Geometry: final body of the model. Coordinates: model frame, mm. Give positions to 0.01 mm unless a question says otherwise; leave off trailing zeros. Write each loop counter-clockwise with the first axis right and the second up, starting at its lowest first coordinate (ties: lowest second). Pieces come first, ordered by that corner, then holes.
Q1. Section A-A (z = -6). Return the cut outline in (x, y), plus the area to 3 significant figures.
Q2. Section B-B (x = -18). Return the cut outline in (y, z), plus the area to 3 significant figures.
Q3. Section C-C (y = -0.35). Return the cut outline in (x, z).
Q4. Pin query (flat end, axial travel): pin 1 Ø4.5 at (x, z) = (-36.5, 36.5) entering from +Y; pin 2 Ø0.8 at (x, y) = (7, -0.5) entering from +Z; pin 3 Ø0.8 at (y, z) = (-0.5, -15.5) entering from +X. Return the tip coordinate at first contact, or that it passes through.
Q5. Line query: line 1 (Z direction, x = 36.5, y = 0.75); line 2 (X direction, y = 0.55, z = -1). Output: solid intervals per line, ascending.
Q6. Section D-D (x = 36.5). Return the cut outline in (y, z), plus the area to 3 significant figures.
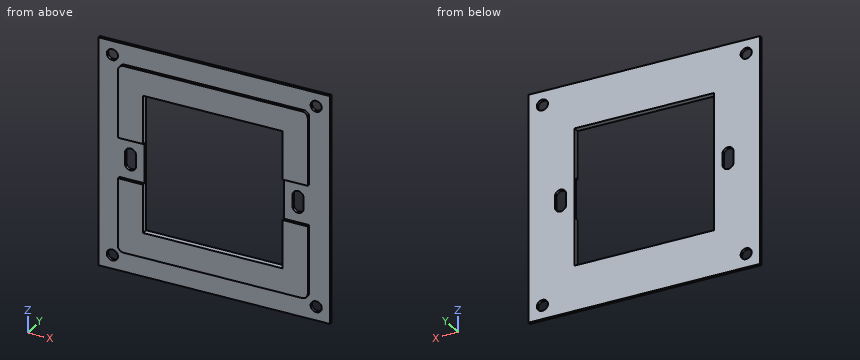
from build123d import *

# Parameters (mm, degrees)
SKETCH_1_W      = 83
SKETCH_1_H      = 83
SKETCH_1_R      = 2
SKETCH_1_W_2    = 50
SKETCH_1_H_2    = 50
EXTRUDE_1_DEPTH = 1
EXTRUDE_2_DEPTH = 1


with BuildPart() as part:
    # Эскиз1 → Бобышка-Вытянуть1 (new body)
    with BuildSketch(Plane(origin=(0, 0, 0), x_dir=(1, 0, 0), z_dir=(0, 1, 0))):
        Rectangle(SKETCH_1_W, SKETCH_1_H)
        with Locations((36.5, 36.5)):
            Circle(SKETCH_1_R, mode=Mode.SUBTRACT)
        with Locations((-36.5, 36.5)):
            Circle(SKETCH_1_R, mode=Mode.SUBTRACT)
        with Locations((-36.5, -36.5)):
            Circle(SKETCH_1_R, mode=Mode.SUBTRACT)
        with Locations((36.5, -36.5)):
            Circle(SKETCH_1_R, mode=Mode.SUBTRACT)
        with BuildLine():
            Line((28, 2), (28, -2))
            ThreePointArc((28, -2), (30, -4), (32, -2))
            Line((32, -2), (32, 2))
            ThreePointArc((32, 2), (30, 4), (28, 2))
        make_face(mode=Mode.SUBTRACT)
        Rectangle(SKETCH_1_W_2, SKETCH_1_H_2, mode=Mode.SUBTRACT)
        with BuildLine():
            Line((-32, 2), (-32, -2))
            ThreePointArc((-32, -2), (-30, -4), (-28, -2))
            Line((-28, -2), (-28, 2))
            ThreePointArc((-28, 2), (-30, 4), (-32, 2))
        make_face(mode=Mode.SUBTRACT)
    extrude(amount=EXTRUDE_1_DEPTH)

    # Эскиз2 → Бобышка-Вытянуть2 (add)
    with BuildSketch(Plane(origin=(0, 0, 0), x_dir=(1, 0, 0), z_dir=(0, 1, 0))):
        with BuildLine():
            Line((-25, -7.393137128), (-34, -7.393137128))
            Line((-34, -7.393137128), (-34, -32))
            ThreePointArc((-34, -32), (-33.414213562, -33.414213562), (-32, -34))
            Line((-32, -34), (32, -34))
            ThreePointArc((32, -34), (33.414213562, -33.414213562), (34, -32))
            Line((34, -32), (34, -7.393137128))
            Line((34, -7.393137128), (25, -7.393137128))
            Line((25, -7.393137128), (25, -25))
            Line((25, -25), (-25, -25))
            Line((-25, -25), (-25, -7.393137128))
        make_face()
        with BuildLine():
            Line((-25, 25), (-25, 7.393137128))
            Line((-25, 7.393137128), (-34, 7.393137128))
            Line((-34, 7.393137128), (-34, 32))
            ThreePointArc((-34, 32), (-33.414213562, 33.414213562), (-32, 34))
            Line((-32, 34), (32, 34))
            ThreePointArc((32, 34), (33.414213562, 33.414213562), (34, 32))
            Line((34, 32), (34, 7.393137128))
            Line((34, 7.393137128), (25, 7.393137128))
            Line((25, 7.393137128), (25, 25))
            Line((25, 25), (-25, 25))
        make_face()
    extrude(amount=-EXTRUDE_2_DEPTH)


solid = part.part
Computed:
1. outline: (-41.5, 0) - (-25, 0) - (-25, 1) - (-41.5, 1) - close; (25, 0) - (41.5, 0) - (41.5, 1) - (25, 1) - close
1. area: 33.0 mm2
2. outline: (-1, -34) - (0, -34) - (0, -41.5) - (1, -41.5) - (1, -25) - (-1, -25) - close; (-1, 25) - (1, 25) - (1, 41.5) - (0, 41.5) - (0, 34) - (-1, 34) - close
2. area: 51.0 mm2
3. outline: (-34, -32) arc R2 ccw to (-32, -34) - (32, -34) arc R2 ccw to (34, -32) - (34, -7.39) - (25, -7.39) - (25, -25) - (-25, -25) - (-25, -7.39) - (-34, -7.39) - close; (-34, 7.39) - (-25, 7.39) - (-25, 25) - (25, 25) - (25, 7.39) - (34, 7.39) - (34, 32) arc R2 ccw to (32, 34) - (-32, 34) arc R2 ccw to (-34, 32) - close
4. pin 1: stops at y = 1
4. pin 2: stops at z = 34
4. pin 3: stops at x = 34
5. line 1: z = -41.5 to -38.5, -34.5 to 34.5, 38.5 to 41.5
5. line 2: x = -41.5 to -32, -28 to -25, 25 to 28, 32 to 41.5
6. outline: (0, -41.5) - (1, -41.5) - (1, -38.5) - (0, -38.5) - close; (0, -34.5) - (1, -34.5) - (1, 34.5) - (0, 34.5) - close; (0, 38.5) - (1, 38.5) - (1, 41.5) - (0, 41.5) - close
6. area: 75.0 mm2
